```python
from build123d import *

# Parameters (mm, degrees)
BOSS_EXTRUDE1_DEPTH = 4.5
SKETCH2_R           = 1.65
BOSS_EXTRUDE2_DEPTH = 3
FILLET1_R           = 10


with BuildPart() as part:
    # Sketch1 → Boss-Extrude1 (new body)
    with BuildSketch(Plane.XY):
        Polygon((145, -50.8), (119.218266921, -36.385786438), (24.218266921, -36.385786438), (0, -50.8), (0, -58.385786438), (2.585786438, -55.8), (142.414213562, -55.8), (145, -58.385786438), align=None)
    extrude(amount=BOSS_EXTRUDE1_DEPTH)

    # Sketch2 → Boss-Extrude2 (add)
    with BuildSketch(Plane(origin=(0, -53.8, 0), x_dir=(1, 0, 0), z_dir=(0, 1, 0))):
        with BuildLine():
            Line((123.505440237, 0), (110.90639088, 12.599049358))
            ThreePointArc((110.90639088, 12.599049358), (109.349158805, 13.639558564), (107.51227833, 14.004936808))
            Line((107.51227833, 14.004936808), (37.48772167, 14.004936808))
            ThreePointArc((37.48772167, 14.004936808), (35.650841195, 13.639558564), (34.09360912, 12.599049358))
            Line((34.09360912, 12.599049358), (21.494559763, 0))
            Line((21.494559763, 0), (123.505440237, 0))
        make_face()
        with Locations((37.48772167, 9.204936808)):
            Circle(SKETCH2_R, mode=Mode.SUBTRACT)
        with Locations((107.51227833, 9.204936808)):
            Circle(SKETCH2_R, mode=Mode.SUBTRACT)
    extrude(amount=BOSS_EXTRUDE2_DEPTH)

    # Fillet1
    fillet1_edges = [part.edges().sort_by_distance(p)[0] for p in [
        (119.218266921, -36.385786438, 2.25),
        (24.218266921, -36.385786438, 2.25),
    ]]
    fillet(fillet1_edges, radius=FILLET1_R)


solid = part.part
```
Geometry check sheet. Reference: the model listing, model coordinates, mm. A direction names the side the tool comes from. Coordinates: 2 decimals unless noted, no trailing zeros. Loops run counter-clockwise (first coordinate to the right, second up) from the corner with the lowest first, then second, coordinate; pieces in that order, holes last. Notation, with made-up numbers: (8.25, -16) - (65.25, -16) arc R29 ccw to (65.25, 13) - close; hole circle Ø2 at (10.25, 66.5). An arc over 180 degrees is marked (long way). One line per item, written item: value. Start each with the question number.
(1) Cross-section at B-B on x = 44. Enter the section's corners in (y, z).
(2) Depth check by flat-ended pin: P1, Ø2, axis at y = -50.5, z = -3, coming from the +X side; P2, Ø11, axis at x = 78.5, z = -4.5, coming from the -Y side; P3, Ø4, axis at x = 107.51, z = -9.2, coming from the +Y side. Enter the tip coordinate at first touch or a pass-through.
(3) Mould release check, pull along X, two halves, no side actions. Record for faces 1 (the cylindrical face through (109.086, -52.321, -9.701)), 2 (the cylindrical face through (119.17, -36.72, 2.28)), 3 (the cylindrical face through (24.353, -36.734, 2.282)): released by +X, released by -X, zero draft, split by the parting line, or undercut.
(4) Tool access check on faces 4 (the flat face through (72, -53.8, -7)), 5 (the flat face through (72, -50.8, -7)), 6 (the flat face through (143.689, -57.075, 2.218)). Record the directions out of +Z, -Z, +X, -X, +Y, -Y that give a thin tool (end or side, any length) a straight path to the whole face; none if there is none.
(5) Cross-section at C-C on y = -48. Enter the section's corners in (x, z).
(6) Material ranges on line 1 (Z direction, x = 115, y = -50); line 2 (Y direction, x = 66.5, z = -2.75); line 3 (Y direction, x = 96.5, z = 2), recorded low to high. Write a range as [from, to].
(7) Cross-section at D-D on x = 112.5. Enter the section's corners in (y, z).
(8) Cross-section at A-A on z = 1.5. Enter the section's corners in (x, y).
Results below:
1. outline: (-55.8, 0) - (-53.8, 0) - (-53.8, -14) - (-50.8, -14) - (-50.8, 0) - (-36.39, 0) - (-36.39, 4.5) - (-55.8, 4.5) - close
2. P1: stops at x = 121.46
2. P2: stops at y = -55.8
2. P3: stops at y = -50.8
3. face 1: undercut
3. face 2: released by +X
3. face 3: released by -X
4. face 4: -Z, +X, -X, -Y
4. face 5: -Z, +X, -X, +Y
4. face 6: +Z, -Z, -Y
5. outline: (4.7, 0) - (139.99, 0) - (139.99, 4.5) - (4.7, 4.5) - close
6. line 1: z = [0, 4.5]
6. line 2: y = [-53.8, -50.8]
6. line 3: y = [-55.8, -36.39]
7. outline: (-55.8, 0) - (-53.8, 0) - (-53.8, -11.01) - (-50.8, -11.01) - (-50.8, 0) - (-36.39, 0) - (-36.39, 4.5) - (-55.8, 4.5) - close
8. outline: (0, -58.39) - (2.59, -55.8) - (142.41, -55.8) - (145, -58.39) - (145, -50.8) - (121.49, -37.66) arc R10 ccw to (116.61, -36.39) - (26.97, -36.39) arc R10 ccw to (21.85, -37.79) - (0, -50.8) - close
